```python
from build123d import *

# Parameters (mm, degrees)
SKETCH1_W           = 58
SKETCH1_H           = 12
SKETCH1_R           = 1.55
BOSS_EXTRUDE1_DEPTH = 6
SKETCH2_W           = 72
SKETCH2_H           = 55
SKETCH2_R           = 1.55
SKETCH2_R_2         = 3.05
BOSS_EXTRUDE2_DEPTH = 4


with BuildPart() as part:
    # Sketch1 → Boss-Extrude1 (new body)
    with BuildSketch(Plane.XY):
        Rectangle(SKETCH1_W, SKETCH1_H)
        with Locations((-19, 0)):
            Circle(SKETCH1_R, mode=Mode.SUBTRACT)
        with Locations((19, 0)):
            Circle(SKETCH1_R, mode=Mode.SUBTRACT)
    extrude(amount=BOSS_EXTRUDE1_DEPTH)

    # Sketch2 → Boss-Extrude2 (add)
    with BuildSketch(Plane.XY.offset(6)):
        with Locations((0, -4)):
            Rectangle(SKETCH2_W, SKETCH2_H)
        with Locations((32.1, 5)):
            Circle(SKETCH2_R, mode=Mode.SUBTRACT)
        with Locations((-20, -28)):
            Circle(SKETCH2_R, mode=Mode.SUBTRACT)
        with Locations((-18.7, 20.2)):
            Circle(SKETCH2_R, mode=Mode.SUBTRACT)
        with Locations((32.1, -22.9)):
            Circle(SKETCH2_R, mode=Mode.SUBTRACT)
        with Locations((-19, 0)):
            Circle(SKETCH2_R_2, mode=Mode.SUBTRACT)
        with Locations((19, 0)):
            Circle(SKETCH2_R_2, mode=Mode.SUBTRACT)
    extrude(amount=BOSS_EXTRUDE2_DEPTH)


solid = part.part
```
Geometry: final body of the model. Coordinates: model frame, mm. A direction names the side the tool comes from. Round coordinates to 2 decimals unless told otherwise and drop trailing zeros. Order: outer loops, then holes, each group sorted by start corner. A loop starts at its lowest first (then second) coordinate and runs counter-clockwise, first axis right, second up. Notation, with made-up numbers: (65, 51) -> (79, 51) arc R19 ccw to (79, 79) -> close; hole circle Ø10 at (74.5, 6). An arc over 180 degrees is marked (long way). Use one line per item in the form item = value. Start each with the question number.
1. Cut plane B-B (y = -28). Return the cut outline in (x, z), then the cut area to 3 significant figures.
2. Cut plane A-A (x = 32.1). Return the cut outline in (y, z).
3. Cut plane C-C (z = 9). Return the cut outline in (x, y).
4. Line query: probe 1 along X at (y, z) = (4, 1.25); probe 2 along Y at (x, z) = (-19, 3.55); probe 3 along Z at (x, y) = (32, 1). Output: solid intervals per line, ascending.
5. Pin query (flat end, axial travel): pin 1 Ø4 at (x, y) = (24, -12) entering from -Z; pin 2 Ø4 at (x, z) = (-3, 1.5) entering from +Y; pin 3 Ø3 at (y, z) = (-2.5, 3) entering from -X. Return the tip coordinate at first contact, or that it passes through.
6. Reachability of faces 1 (the face through (-29, 0, 3)), 2 (the face through (-17.7, -1.3, 6)), 3 (the face through (0, 6, 3)) from +Z, -Z, +X, -X, +Y, -Y: full face, straight path, thin tool, end or side. Return the list, or none.
7. Cut plane D-D (x = 19). Return the cut outline in (y, z).
8. Draft query along X for faces 4 (the face through (20.432, -0.594, 2.958)), 5 (the face through (33.578, -22.434, 7.972)), 6 (the face through (-1, 23.5, 8)), 7 (the face through (29, 0, 3)). Return one class per face: pulls with the +X half, pulls with the -X half, needs draft (parallel to the pull), parting line crosses it, or undercut.
Solution:
q1.outline = (-36, 6) -> (-21.55, 6) -> (-21.55, 10) -> (-36, 10) -> close; (-18.45, 6) -> (36, 6) -> (36, 10) -> (-18.45, 10) -> close
q1.area = 276 mm^2
q2.outline = (-31.5, 6) -> (-24.45, 6) -> (-24.45, 10) -> (-31.5, 10) -> close; (-21.35, 6) -> (3.45, 6) -> (3.45, 10) -> (-21.35, 10) -> close; (6.55, 6) -> (23.5, 6) -> (23.5, 10) -> (6.55, 10) -> close
q3.outline = (-36, -31.5) -> (36, -31.5) -> (36, 23.5) -> (-36, 23.5) -> close; hole circle Ø6.1 at (-19, 0); hole circle Ø3.1 at (-20, -28); hole circle Ø3.1 at (-18.7, 20.2); hole circle Ø6.1 at (19, 0); hole circle Ø3.1 at (32.1, -22.9); hole circle Ø3.1 at (32.1, 5)
q4.probe_1 = -29 to 29
q4.probe_2 = -6 to -1.55, 1.55 to 6
q4.probe_3 = 6 to 10
q5.pin_1 = 6
q5.pin_2 = 6
q5.pin_3 = -29
q6.face_1 = -Z, -X, +Y, -Y
q6.face_2 = +Z
q6.face_3 = -Z, +X, -X, +Y
q7.outline = (-31.5, 6) -> (-6, 6) -> (-6, 0) -> (-1.55, 0) -> (-1.55, 6) -> (-3.05, 6) -> (-3.05, 10) -> (-31.5, 10) -> close; (1.55, 0) -> (6, 0) -> (6, 6) -> (23.5, 6) -> (23.5, 10) -> (3.05, 10) -> (3.05, 6) -> (1.55, 6) -> close
q8.face_4 = undercut
q8.face_5 = undercut
q8.face_6 = needs draft
q8.face_7 = pulls with the +X half
